```python
from build123d import *

# Parameters (mm, degrees)
SKETCH2_W           = 203.2
SKETCH2_H           = 6.35
SKETCH2_R           = 1.5875
BOSS_EXTRUDE1_DEPTH = 31.75
SKETCH4_W           = 6.35
SKETCH4_H           = 19.05
BOSS_EXTRUDE2_DEPTH = 50.8
SKETCH6_W           = 12.7
SKETCH6_H           = 3.175
CUT_EXTRUDE1_DEPTH  = 32.75


with BuildPart() as part:
    # Sketch2 → Boss-Extrude1 (new body)
    with BuildSketch(Plane(origin=(0, 0, 0), x_dir=(1, 0, 0), z_dir=(0, 1, 0))):
        Rectangle(SKETCH2_W, SKETCH2_H)
        with Locations((-76.2, 0)):
            Circle(SKETCH2_R, mode=Mode.SUBTRACT)
        with Locations((-44.45, 0)):
            Circle(SKETCH2_R, mode=Mode.SUBTRACT)
        with Locations((-12.7, 0)):
            Circle(SKETCH2_R, mode=Mode.SUBTRACT)
        with Locations((19.05, 0)):
            Circle(SKETCH2_R, mode=Mode.SUBTRACT)
        with Locations((50.8, 0)):
            Circle(SKETCH2_R, mode=Mode.SUBTRACT)
        with Locations((82.55, 0)):
            Circle(SKETCH2_R, mode=Mode.SUBTRACT)
    boss_extrude1 = extrude(amount=BOSS_EXTRUDE1_DEPTH)

    # Sketch4 → Boss-Extrude2 (add)
    with BuildSketch(Plane.XY.offset(3.175)):
        with Locations((-98.425, 22.225)):
            Rectangle(SKETCH4_W, SKETCH4_H)
    extrude(amount=BOSS_EXTRUDE2_DEPTH)

    # Mirror1: Boss-Extrude1 across plane
    add(boss_extrude1.mirror(Plane.XY.offset(28.575)))

    # Sketch6 → Cut-Extrude1 (cut, through all)
    with BuildSketch(Plane(origin=(0, 31.75, 0), x_dir=(1, 0, 0), z_dir=(0, 1, 0))):
        with Locations((95.25, 1.5875)):
            Rectangle(SKETCH6_W, SKETCH6_H)
        with Locations((95.25, -58.7375)):
            Rectangle(SKETCH6_W, SKETCH6_H)
    extrude(amount=-CUT_EXTRUDE1_DEPTH, mode=Mode.SUBTRACT)


solid = part.part
```
Input: part model. Units: mm. Frame: model coordinates. A direction names the side the tool comes from. Coordinates: 2 decimals unless noted, no trailing zeros. Write each loop counter-clockwise with the first axis right and the second up, starting at its lowest first coordinate (ties: lowest second). Pieces come first, ordered by that corner, then holes. Notation, with made-up numbers: M 47.25,-36 L 76.25,-36 A26 cw 76.25,-6 Z; hole C 54.25,35 d10. An arc over 180 degrees is marked long. Use one line per item in the form item = value.
Q1. Draft query along Z for faces 1 (the face through (-1, 16, 3.175)), 2 (the face through (-16, 31.75, 3)), 3 (the face through (95, 16, 0)), 4 (the face through (-8, 16, 60.325)). Return one class per face: released by +Z, released by -Z, zero draft, split by the parting line, or undercut.
Answer below:
face_1 = undercut
face_2 = zero draft
face_3 = released by -Z
face_4 = released by +Z
Q2. Set-up query: faces 5 (the face through (95, 16, 57.15)), 6 (the face through (-95.25, 22, 28)), 7 (the face through (-98, 12.7, 28)), 8 (the face through (-101.6, 19, 28)), 9 (the face through (-8, 16, -3.175)). Return all of +Z, -Z, +X, -X, +Y, -Y with unobstructed straight access to the full face (end or side cutting, diameter ignored); none if empty.
Answer below:
face_5 = +Z, +X, +Y, -Y
face_6 = +X, +Y, -Y
face_7 = +X, -X, -Y
face_8 = +Z, -Z, -X, +Y, -Y
face_9 = -Z, +X, -X, +Y, -Y
Q3. Section A-A (x = 70). Return loops of the section in (y, z) (3 decimals), plus the area to 3 significant figures.
Answer below:
outline = M 0,-3.175 L 31.75,-3.175 L 31.75,3.175 L 0,3.175 Z; M 0,53.975 L 31.75,53.975 L 31.75,60.325 L 0,60.325 Z
area = 403 mm²
Q4. Section B-B (y = 10). Count the separate pieces of the cut face and the enclosed holes in it, plus the area to 3 significant figures.
Answer below:
separate_pieces = 2
enclosed_holes = 12
area = 2,400 mm²
Q5. Material intervals for probe 1 along Z at (x, y) = (-76, 9) (3 decimals); probe 2 along Z at (x, y) = (-48.5, 18.5) (3 decimals); probe 3 along Z at (x, y) = (89, 13.5) (3 decimals), sorted ascending. Write a range as from..to.
Answer below:
probe_1 = -3.175..-1.575, 1.575..3.175, 53.975..55.575, 58.725..60.325
probe_2 = -3.175..3.175, 53.975..60.325
probe_3 = 0..3.175, 53.975..57.15
Q6. First-contact query: pin 1 (2.5 mm diameter, centred on x = 19.05, z = 57.15, fed in from +Y); pin 2 (1 mm diameter, centred on y = 10.5, z = 59.5, fed in from +X); pin 3 (5 mm diameter, centred on x = -97.5, z = 27.5, fed in from -Y); pin 4 (4 mm diameter, centred on x = 96.5, y = 8.5, fed in from -Z). Flat tips, straight axial feed; report the tip coordinate or a pass-through.
Answer below:
pin_1 = through
pin_2 = 88.9
pin_3 = 12.7
pin_4 = 0
